Could you check a few things on this drawing? It's one solid part, dimensions in mm from its lowest x, y, z. A direction names the side the tool comes from. Round coordinates to 2 decimals unless told otherwise and drop trailing zeros. Loops run counter-clockwise (first coordinate to the right, second up) from the corner with the lowest first, then second, coordinate; pieces in that order, holes last. Notation, with made-up numbers: (4.5, 39.5) -> (46.5, 39.5) arc R18 ccw to (46.5, 54.5) -> close; hole circle Ø11 at (-29.5, 2.25). An arc over 180 degrees is marked (long way). Use one line per item in the form item = value. Start each with the question number.
Item 1: If we section it at B-B (x = 10): Write out the boundary of the cut face in (y, z).
Item 2: If we section it at D-D (y = 22): Write out the boundary of the cut face in (x, z).
Item 3: If we section it at C-C (x = 1.25): Write out the boundary of the cut face in (y, z).
Item 4: I'm going to push flat-ended pins straight in: pin 1 Ø1.2 at (x, z) = (18, 1.5) entering from +Y; pin 2 Ø1.2 at (x, z) = (17.5, 2) entering from -Y; pin 3 Ø2.5 at (x, y) = (10, 27.5) entering from -Z. Where does each tip first touch, or does it pass through?
Item 5: For the marked faces 1, 2, 3 and 4, which set-ups out of +Z, -Z, +X, -X, +Y, -Y let a thin tool reach every point of the face, with its end or its side?
Item 6: Thinking about a two-plate mould opening in X: for the marked faces 5, 6, 7 and 8, which applies, released by +X, released by -X, zero draft, split by the parting line, or undercut?
Item 7: If I drill on L1, parallel to Y at x = 10, z = 2.1; L2, parallel to X at y = 3, z = 2.95; L3, parallel to X at y = 20, z = 2.8, over which ranges is the centre line in solid material (lowest first)? Write a range as [from, to].
Item 8: If we section it at A-A (z = 0.75): Write out the boundary of the cut face in (x, y).
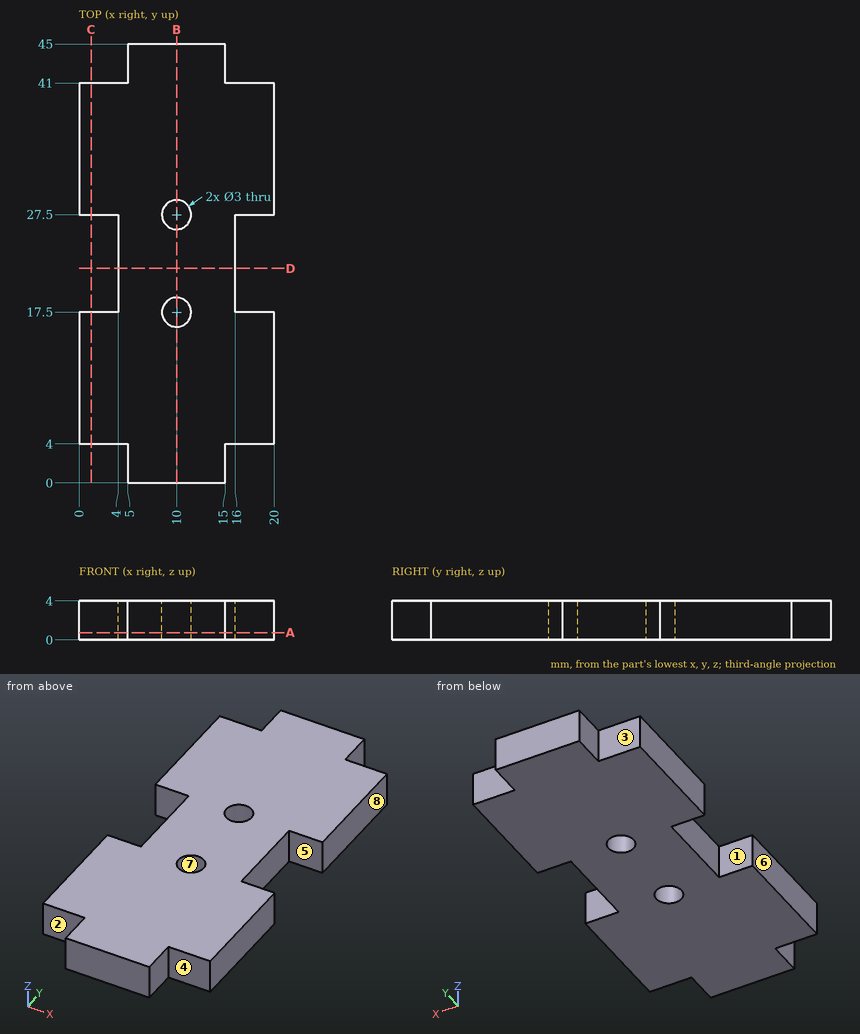
Values found:
q1.outline = (0, 0) -> (16, 0) -> (16, 4) -> (0, 4) -> close; (19, 0) -> (26, 0) -> (26, 4) -> (19, 4) -> close; (29, 0) -> (45, 0) -> (45, 4) -> (29, 4) -> close
q2.outline = (4, 0) -> (16, 0) -> (16, 4) -> (4, 4) -> close
q3.outline = (4, 0) -> (17.5, 0) -> (17.5, 4) -> (4, 4) -> close; (27.5, 0) -> (41, 0) -> (41, 4) -> (27.5, 4) -> close
q4.pin_1 = 41
q4.pin_2 = 4
q4.pin_3 = through
q5.face_1 = +Z, -Z, -X
q5.face_2 = +Z, -Z, -X, -Y
q5.face_3 = +Z, -Z, -X, +Y
q5.face_4 = +Z, -Z, +X, -Y
q6.face_5 = zero draft
q6.face_6 = released by -X
q6.face_7 = undercut
q6.face_8 = released by +X
q7.L1 = [0, 16], [19, 26], [29, 45]
q7.L2 = [5, 15]
q7.L3 = [4, 16]
q8.outline = (0, 4) -> (5, 4) -> (5, 0) -> (15, 0) -> (15, 4) -> (20, 4) -> (20, 17.5) -> (16, 17.5) -> (16, 27.5) -> (20, 27.5) -> (20, 41) -> (15, 41) -> (15, 45) -> (5, 45) -> (5, 41) -> (0, 41) -> (0, 27.5) -> (4, 27.5) -> (4, 17.5) -> (0, 17.5) -> close; hole circle Ø3 at (10, 17.5); hole circle Ø3 at (10, 27.5)
